```python
from build123d import *

# Parameters (mm, degrees)
SKETCH1_W                = 1600
SKETCH1_H                = 1600
BOSS_EXTRUDE1_DEPTH      = 25
SKETCH2_W                = 1600
SKETCH2_H                = 1100
SKETCH2_W_2              = 1550
SKETCH2_H_2              = 1050
BOSS_EXTRUDE2_DEPTH      = 1100
BOSS_EXTRUDE3_DEPTH      = 50
BOSS_EXTRUDE3_DEPTH_BACK = 1650
CUT_EXTRUDE1_DEPTH       = 2648.749751348
BOSS_EXTRUDE4_DEPTH      = 12.5
BOSS_EXTRUDE5_DEPTH      = 67.5
SKETCH8_W                = 400
SKETCH8_H                = 650
SKETCH8_W_2              = 350
SKETCH8_H_2              = 350
CUT_EXTRUDE2_DEPTH       = 68.5
SKETCH9_W                = 510
SKETCH9_H                = 510
SKETCH9_W_2              = 350
SKETCH9_H_2              = 350
BOSS_EXTRUDE6_DEPTH      = 10
BOSS_EXTRUDE7_REACH      = 2638.073
SKETCH10_W               = 50
SKETCH10_H               = 50
SCALE1_SCALE             = 0.125
SCALE2_SCALE             = 0.5
BOSS_EXTRUDE9_DEPTH      = 101


with BuildPart() as part:
    # Sketch1 → Boss-Extrude1 (new body)
    with BuildSketch(Plane(origin=(0, 0, 0), x_dir=(1, 0, 0), z_dir=(0, 1, 0))):
        with Locations((800, 800)):
            Rectangle(SKETCH1_W, SKETCH1_H)
    extrude(amount=BOSS_EXTRUDE1_DEPTH)

    # Sketch2 → Boss-Extrude2 (add)
    with BuildSketch(Plane(origin=(0, 25, 0), x_dir=(1, 0, 0), z_dir=(0, 1, 0))):
        with Locations((800, 1050)):
            Rectangle(SKETCH2_W, SKETCH2_H)
        with Locations((800, 1050)):
            Rectangle(SKETCH2_W_2, SKETCH2_H_2, mode=Mode.SUBTRACT)
    extrude(amount=BOSS_EXTRUDE2_DEPTH)

    # Sketch3 → Boss-Extrude3 (add, two sides: drawn at the far end of the back side and taken through both)
    with BuildSketch(Plane(origin=(1600, 0, 0), x_dir=(0, 0, -1), z_dir=(1, 0, 0)).offset(-BOSS_EXTRUDE3_DEPTH_BACK)):
        Polygon((1600, 925), (500, 1125), (-32.556177987, 1221.828395998), (-28.084042032, 1246.42514375), (1653.633304815, 940.474679295), (1649.193495505, 916.05572809), align=None)
    extrude(amount=BOSS_EXTRUDE3_DEPTH + BOSS_EXTRUDE3_DEPTH_BACK)

    # Sketch4 → Cut-Extrude1 (cut, through all)
    with BuildSketch(Plane(origin=(1600, 0, 0), x_dir=(0, 0, -1), z_dir=(1, 0, 0))):
        Polygon((-28.084042032, 1246.42514375), (1653.633304815, 940.474679295), (1653.633304815, 1246.42514375), align=None)
    extrude(amount=-CUT_EXTRUDE1_DEPTH, mode=Mode.SUBTRACT)

    # Sketch5 → Boss-Extrude4 (add)
    with BuildSketch(Plane(origin=(1600, 0, 0), x_dir=(0, 0, -1), z_dir=(1, 0, 0))):
        Polygon((1532.5, 937.272727273), (1532.5, 0), (1612.5, 0), (1612.5, 922.727272727), align=None)
        Polygon((567.5, 1112.727272727), (567.5, 0), (487.5, 0), (487.5, 1127.272727273), align=None)
    boss_extrude4 = extrude(amount=BOSS_EXTRUDE4_DEPTH)

    # Sketch6 → Boss-Extrude5 (add)
    with BuildSketch(Plane.ZY.offset(-1600)):
        Polygon((-1600, 925), (-1600, 0), (-1612.5, 0), (-1612.5, 922.727272727), align=None)
        Polygon((-487.5, 1127.272727273), (-500, 1125), (-500, 25), (-487.5, 25), align=None)
    boss_extrude5 = extrude(amount=BOSS_EXTRUDE5_DEPTH)

    # Mirror1: Boss-Extrude4, Boss-Extrude5 across plane
    add(boss_extrude4.mirror(Plane(origin=(800, 0, 0), x_dir=(0, 0, 1), z_dir=(1, 0, 0))))
    add(boss_extrude5.mirror(Plane(origin=(800, 0, 0), x_dir=(0, 0, 1), z_dir=(1, 0, 0))))

    # Sketch8 → Cut-Extrude2 (cut)
    with BuildSketch(Plane.XY.offset(-500)):
        with Locations((400, 350)):
            Rectangle(SKETCH8_W, SKETCH8_H)
        with Locations((1175, 550)):
            Rectangle(SKETCH8_W_2, SKETCH8_H_2)
    extrude(amount=-CUT_EXTRUDE2_DEPTH, mode=Mode.SUBTRACT)

    # Sketch9 → Boss-Extrude6 (add)
    # profile 1 of 2: a face of its own
    with BuildSketch(Plane.XY.offset(-500)):
        Polygon((200, 25), (200, 673.570628699), (200, 675), (600, 675), (600, 673.570628699), (600, 25), (680, 25), (680, 753.570628699), (120, 753.570628699), (120, 25), align=None)
    # profile 2 of 2: a face of its own
    with BuildSketch(Plane.XY.offset(-500)):
        with Locations((1175, 550)):
            Rectangle(SKETCH9_W, SKETCH9_H)
        with Locations((1175, 550)):
            Rectangle(SKETCH9_W_2, SKETCH9_H_2, mode=Mode.SUBTRACT)
    extrude(amount=BOSS_EXTRUDE6_DEPTH)

    # Boss-Extrude7: up to this plane
    boss_extrude7_end = Plane(origin=(1650, 925, -1600), z_dir=(0, 0.9838699100999074, -0.1788854381999831))
    # Sketch10 → Boss-Extrude7 (add, up to the surface)
    with BuildSketch(Plane(origin=(0, 25, 0), x_dir=(1, 0, 0), z_dir=(0, 1, 0)), mode=Mode.PRIVATE) as boss_extrude7_sk1:
        with Locations((50, 1550)):
            Rectangle(SKETCH10_W, SKETCH10_H)
    boss_extrude7_tool1 = split(extrude(boss_extrude7_sk1.sketch, amount=BOSS_EXTRUDE7_REACH, mode=Mode.PRIVATE), bisect_by=boss_extrude7_end, keep=Keep.BOTH, mode=Mode.PRIVATE)
    add(boss_extrude7_tool1.solids().sort_by_distance((50, 25, -1550))[0])
    # Sketch10 → Boss-Extrude7 (add, up to the surface)
    with BuildSketch(Plane(origin=(0, 25, 0), x_dir=(1, 0, 0), z_dir=(0, 1, 0)), mode=Mode.PRIVATE) as boss_extrude7_sk2:
        with Locations((1550, 1550)):
            Rectangle(SKETCH10_W, SKETCH10_H)
    boss_extrude7_tool2 = split(extrude(boss_extrude7_sk2.sketch, amount=BOSS_EXTRUDE7_REACH, mode=Mode.PRIVATE), bisect_by=boss_extrude7_end, keep=Keep.BOTH, mode=Mode.PRIVATE)
    add(boss_extrude7_tool2.solids().sort_by_distance((1550, 25, -1550))[0])
    # Sketch10 → Boss-Extrude7 (add, up to the surface)
    with BuildSketch(Plane(origin=(0, 25, 0), x_dir=(1, 0, 0), z_dir=(0, 1, 0)), mode=Mode.PRIVATE) as boss_extrude7_sk3:
        with Locations((50, 550)):
            Rectangle(SKETCH10_W, SKETCH10_H)
    boss_extrude7_tool3 = split(extrude(boss_extrude7_sk3.sketch, amount=BOSS_EXTRUDE7_REACH, mode=Mode.PRIVATE), bisect_by=boss_extrude7_end, keep=Keep.BOTH, mode=Mode.PRIVATE)
    add(boss_extrude7_tool3.solids().sort_by_distance((50, 25, -550))[0])
    # Sketch10 → Boss-Extrude7 (add, up to the surface)
    with BuildSketch(Plane(origin=(0, 25, 0), x_dir=(1, 0, 0), z_dir=(0, 1, 0)), mode=Mode.PRIVATE) as boss_extrude7_sk4:
        with Locations((1550, 550)):
            Rectangle(SKETCH10_W, SKETCH10_H)
    boss_extrude7_tool4 = split(extrude(boss_extrude7_sk4.sketch, amount=BOSS_EXTRUDE7_REACH, mode=Mode.PRIVATE), bisect_by=boss_extrude7_end, keep=Keep.BOTH, mode=Mode.PRIVATE)
    add(boss_extrude7_tool4.solids().sort_by_distance((1550, 25, -550))[0])
    # Sketch10 → Boss-Extrude7 (add, up to the surface)
    with BuildSketch(Plane(origin=(0, 25, 0), x_dir=(1, 0, 0), z_dir=(0, 1, 0)), mode=Mode.PRIVATE) as boss_extrude7_sk5:
        Polygon((725, 525), (750, 525), (800, 525), (800, 575), (750, 575), (750, 1125), (800, 1125), (800, 1175), (750, 1175), (725, 1175), align=None)
    boss_extrude7_tool5 = split(extrude(boss_extrude7_sk5.sketch, amount=BOSS_EXTRUDE7_REACH, mode=Mode.PRIVATE), bisect_by=boss_extrude7_end, keep=Keep.BOTH, mode=Mode.PRIVATE)
    add(boss_extrude7_tool5.solids().sort_by_distance((746.323529, 25, -850))[0])


with BuildPart() as part_1:
    # Scale1: scaled about (0, 0, 0)
    add(part.part.scale(SCALE1_SCALE))


with BuildPart() as part_2:
    # Scale2: scaled about (0, 0, 0)
    add(part_1.part.scale(SCALE2_SCALE))

    # Sketch11 → Boss-Extrude9 (add)
    with BuildSketch(Plane.XY):
        Polygon((0, 0), (100, 0), (100, -20.901409281), align=None)
    extrude(amount=-BOSS_EXTRUDE9_DEPTH)


solid = part_2.part
```
Source: CAD feature listing. Evaluate the final solid. Frame: model axes, mm. A direction names the side the tool comes from. Round coordinates to 2 decimals unless told otherwise and drop trailing zeros. Loops run counter-clockwise (first coordinate to the right, second up) from the corner with the lowest first, then second, coordinate; pieces in that order, holes last. Notation, with made-up numbers: M -16,13 L 30,13 A27 cw 30,45 Z; hole C 44.25,84.25 d9. An arc over 180 degrees is marked long. Use a Markdown table: item, result. Add a question column.
1. Section query B-B on y = 65. Give the number of separate pieces and of enclosed holes in the cut face, then the cut area to 3 significant figures.
2. Contact query for flat-ended pins moving along their axis: P1, Ø3, axis at y = 2.5, z = -73.5, coming from the +X side; P2, Ø16, axis at x = 75, y = 29, coming from the +Z side (3 decimals); P3, Ø0.5, axis at x = 68, z = -100.5, coming from the +Y side. Output: stop coordinate, or through.
3. Section query C-C on z = -18.5. Return the cut outline in (x, y) (1 decimal), then the cut area to 3 significant figures.
4. Line query: line 1 (X direction, y = 35, z = -67.5) (1 decimal); line 2 (Z direction, x = 59.5, y = 57); line 3 (X direction, y = 9.5, z = -33.5). Output: solid intervals per line, ascending.
5. Section query A-A on z = -83.5. Return the cut outline in (x, y) (1 decimal), then the cut area to 3 significant figures.
6. Mould query, pull axis X, two halves, no side actions, for faces 1 (the flat face through (48, 32, -70.312)), 2 (the flat face through (98, 28, -100.781)), 3 (the flat face through (-3.125, 68, -51)). Classes: pulls with the +X half, pulls with the -X half, needs draft (parallel to the pull), parting line crosses it, or undercut.
7. Reachability of faces 4 (the flat face through (62, -7, 0)), 5 (the flat face through (50, 32, -72)), 6 (the flat face through (12, 29, -30.625)) from +Z, -Z, +X, -X, +Y, -Y: full face, straight path, thin tool, end or side. Return the list, or none.
Reported:
| question | item | result |
|---|---|---|
| 1 | separate pieces | 1 |
| 1 | enclosed holes | 2 |
| 1 | area | 1,250 mm² |
| 2 | P1 | stops at x = 100 |
| 2 | P2 | stops at z = -30.625 |
| 2 | P3 | stops at y = 59.34 |
| 3 | outline | M -3.1,72.6 L 103.1,72.6 L 103.1,74.2 L -3.1,74.2 Z; M 0,0 L 100,-20.9 L 100,1.6 L 0,1.6 Z |
| 3 | area | 1,370 mm² |
| 4 | line 1 | x = 0 to 1.6, 45.3 to 46.9, 98.4 to 100 |
| 4 | line 2 | z = -100 to -98.44, -32.81 to -31.25 |
| 4 | line 3 | x = -0.78 to 4.69, 45.31 to 50, 95.31 to 100.78 |
| 5 | outline | M -3.1,60.8 L 0,60.8 L 0,0 L 100,-20.9 L 100,60.8 L 103.1,60.8 L 103.1,62.4 L -3.1,62.4 Z; hole M 1.6,1.6 L 98.4,1.6 L 98.4,60.8 L 1.6,60.8 Z |
| 5 | area | 1,550 mm² |
| 6 | face 1 | undercut |
| 6 | face 2 | needs draft |
| 6 | face 3 | pulls with the -X half |
| 7 | face 4 | +Z, +X, -X, -Y |
| 7 | face 5 | none |
| 7 | face 6 | +Z |
